```python
from build123d import *
from build123d.topology import SkipClean

# Parameters (mm, degrees)
SKETCH2_R           = 9.525
EXTRUDE1_DEPTH      = 17.526
SKETCH15_R          = 11.1125
BOSS_EXTRUDE1_DEPTH = 18.9865
SKETCH16_R          = 4.9657
CUT_EXTRUDE1_DEPTH  = 40.750949281
SKETCH20_R          = 11.1125
BOSS_EXTRUDE2_DEPTH = 18.9865
SKETCH22_R          = 10.668
BOSS_EXTRUDE3_DEPTH = 17.12976
BOSS_EXTRUDE3_TAPER = 1.75
CHAMFER1_SIZE       = 1.360714286
CHAMFER1_SIZE_2     = 1.404253042
SKETCH25_R          = 10.668
BOSS_EXTRUDE4_DEPTH = 17.12976
BOSS_EXTRUDE4_DRAFT = -15
SKETCH28_R          = 7.978385455
CUT_EXTRUDE6_DEPTH  = 17.12976
FILLET1_R           = 0.762
CIRPATTERN1_COUNT   = 2
CIRPATTERN1_ANGLE   = 180
SKETCH26_R          = 4.9657
CUT_EXTRUDE4_DEPTH  = 83.22239678
SKETCH29_R          = 4.9657
CUT_EXTRUDE7_DEPTH  = 53.545547444


with BuildPart() as part:
    # Sketch2 → Extrude1 (new body)
    with BuildSketch(Plane(origin=(-36.5125, 0, 0), x_dir=(0, 0, -1), z_dir=(1, 0, 0))):
        Circle(SKETCH2_R)
    extrude(amount=EXTRUDE1_DEPTH)

    # Sketch5 → Cut-Revolve1 (revolve, cut)
    with BuildSketch(Plane.XY):
        Polygon((-32.818891687, 8.493888504), (-29.643891687, 8.493888504), (-28.612780191, 9.525), (-36.5125, 9.525), (-36.5125, 5.710555), align=None)
        Polygon((-18.9865, 8.493888504), (-20.574, 8.493888504), (-21.605111496, 9.525), (-18.9865, 9.525), align=None)
    revolve(axis=Axis((0, 0, 0), (-1, 0, 0)), mode=Mode.SUBTRACT)

    # Sketch15 → Boss-Extrude1 (add)
    with BuildSketch(Plane(origin=(-18.9865, 0, 0), x_dir=(0, 0, -1), z_dir=(1, 0, 0))):
        Circle(SKETCH15_R)
    extrude(amount=BOSS_EXTRUDE1_DEPTH)

    # Sketch16 → Cut-Extrude1 (cut, through all)
    with BuildSketch(Plane(origin=(0, 0, 0), x_dir=(0, 0, -1), z_dir=(1, 0, 0))):
        Circle(SKETCH16_R)
    extrude(amount=-CUT_EXTRUDE1_DEPTH, mode=Mode.SUBTRACT)

    # Fillet1
    fillet1_edges = [part.edges().sort_by_distance(p)[0] for p in [
        (-18.9865, 0, 11.1125),
    ]]
    fillet(fillet1_edges, radius=FILLET1_R)


with BuildPart() as body_2:
    # Sketch20 → Boss-Extrude2 (new body)
    with BuildSketch(Plane(origin=(0, 18.9865, 0), x_dir=(-1, 0, 0), z_dir=(0, 1, 0))):
        with Locations(Location((0, 0, 0), (0, 0, 90))):
            Circle(SKETCH20_R)
    extrude(amount=-BOSS_EXTRUDE2_DEPTH)


with BuildPart() as body_3:
    # Sketch22 → Boss-Extrude3 (new body)
    with BuildSketch(Plane(origin=(0, 18.9865, 0), x_dir=(-1, 0, 0), z_dir=(0, 1, 0))):
        Circle(SKETCH22_R)
    extrude(amount=BOSS_EXTRUDE3_DEPTH, taper=BOSS_EXTRUDE3_TAPER)

    # Chamfer1
    # the kernel refuses this chamfer: 1.404253042, 1.360714286 mm, written as the material it takes off along each edge
    with BuildSketch(Plane(origin=(0, 36.11626, 0), x_dir=(-1, 0, 0), z_dir=(0, 0, 1))) as chamfer1_piece_1:
        Polygon((10.144638497 + CHAMFER1_SIZE * 0.0305385132034, CHAMFER1_SIZE * 0.999533590627), (10.144638497 - CHAMFER1_SIZE_2, 0), (10.144638497, 0), align=None)
    revolve(axis=Axis((0, 36.11626, 0), (0, -1, 0)), mode=Mode.SUBTRACT)


with BuildPart() as boss_extrude4_tool:
    # Sketch25 → Boss-Extrude4 (with draft: the straight prism first)
    with BuildSketch(Plane.XZ.offset(-18.9865)):
        Circle(SKETCH25_R)
    extrude(amount=-BOSS_EXTRUDE4_DEPTH)
    # Boss-Extrude4: the draft: its side faces are tilted about the plane it starts from
    boss_extrude4_sides = [boss_extrude4_tool.faces().sort_by_distance(p)[0] for p in [
        (-10.668, 27.55138, 0),
    ]]
    draft(boss_extrude4_sides, Plane.XZ.offset(-18.9865), BOSS_EXTRUDE4_DRAFT)


with BuildPart() as body_3_1:
    add(body_3.part)

    # Boss-Extrude4: add boss_extrude4_tool
    add(boss_extrude4_tool.part)

    # Sketch28 → Cut-Extrude6 (cut)
    with BuildSketch(Plane(origin=(0, 36.11626, 0), x_dir=(1, 0, 0), z_dir=(0, 1, 0))):
        with Locations(Location((0, 0, 0), (0, 0, 270))):
            Circle(SKETCH28_R)
    extrude(amount=-CUT_EXTRUDE6_DEPTH, mode=Mode.SUBTRACT)


with BuildPart() as cirpattern1_1:
    # CirPattern1: pattern copy
    add(part.part.rotate(Axis((0, 0, 12.651043997), (0, 0, -1)), 1 * CIRPATTERN1_ANGLE / (CIRPATTERN1_COUNT - 1)))


with BuildPart() as part_1:
    add(part.part)

    # Combine2: union body 3, body 2, CirPattern1_1
    add(body_3_1.part)
    add(body_2.part)
    add(cirpattern1_1.part)

    # Sketch30 → Revolve1 (revolve)
    with SkipClean():  # the faces are left unmerged after this step: merging them gives an invalid solid
        with BuildSketch(Plane.XY, mode=Mode.PRIVATE) as revolve1_sk:
            with BuildLine():
                Line((0, 18.9865), (0, 9.49325))
                ThreePointArc((0, 9.49325), (-5.981989992, 13.352586812), (-10.922, 18.4785))
                Line((-10.922, 18.4785), (-10.922, 18.9865))
                Line((-10.922, 18.9865), (0, 18.9865))
            make_face()
        revolve(revolve1_sk.sketch.rotate(Axis((0, 18.9865, 0), (0, -1, 0)), 270), axis=Axis((0, 18.9865, 0), (0, -1, 0)))

    # Sketch26 → Cut-Extrude4 (cut, through all)
    with SkipClean():  # the faces are left unmerged after this step: merging them gives an invalid solid
        with BuildSketch(Plane.ZY.offset(36.5125)):
            with Locations(Location((0, 0, 0), (0, 0, 180))):
                Circle(SKETCH26_R)
        extrude(amount=-CUT_EXTRUDE4_DEPTH, mode=Mode.SUBTRACT)

    # Sketch29 → Cut-Extrude7 (cut, through all)
    with SkipClean():  # the faces are left unmerged after this step: merging them gives an invalid solid
        with BuildSketch(Plane(origin=(0, 0, 0), x_dir=(1, 0, 0), z_dir=(0, 1, 0))):
            with Locations(Location((0, 0, 0), (0, 0, 270))):
                Circle(SKETCH29_R)
        extrude(amount=CUT_EXTRUDE7_DEPTH, mode=Mode.SUBTRACT)


solid = part_1.part
```
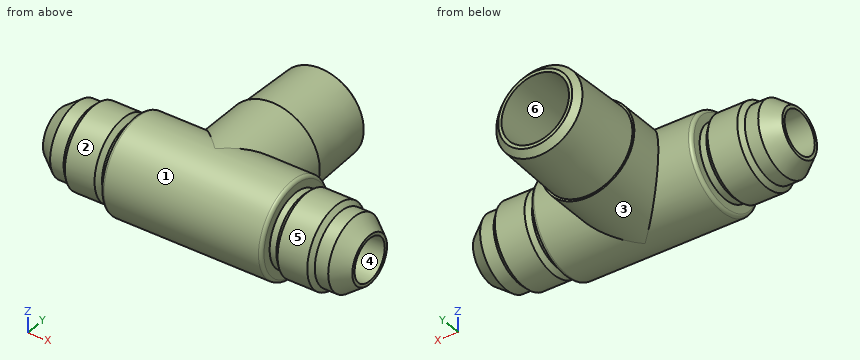
Source: CAD feature listing. Evaluate the final solid. Frame: model axes, mm. Face numbers are marked on the shaded views. A direction names the side the tool comes from. Give positions to 0.01 mm unless a question says otherwise; leave off trailing zeros. Write each loop counter-clockwise with the first axis right and the second up, starting at its lowest first coordinate (ties: lowest second). Pieces come first, ordered by that corner, then holes.
1. Pull-direction query (Y, two-part tool) for the marked faces 4, 5 and 6; classes: +Y half, -Y half, draft (parallel to the pull), parting line (faces both ways), or undercut.
2. Section query C-C (x = 15). Return the cut outline in (y, z) (1 decimal).
3. Section query A-A (x = 0). Return the cut outline in (y, z) (1 decimal).
4. Access query for the marked faces 1, 2 and 3. Directions: +Z, -Z, +X, -X, +Y, -Y. A direction counts if a zero-diameter tool reaches every point of the face in a straight line with its end or side. Return the directions, or none.
5. Section query B-B (z = 0). Count the separate pieces of the cut face and the enclosed holes in it, then the cut area to 3 significant figures.
6. First-contact query: pin 1 (2 mm diameter, centred on y = 28, z = 2.5, fed in from -X); pin 2 (2 mm diameter, centred on x = 16.5, z = -1, fed in from +Y); pin 3 (1 mm diameter, centred on x = -5.5, z = 1.5, fed in from +Y). Flat tips, straight axial feed; report the tip coordinate or a pass-through.
7. Material intervals for line 1 along X through (y, z) = (13.25, 0), sorted ascending.
Output values:
1. face 4: undercut
1. face 5: parting line
1. face 6: draft
2. outline: circle Ø22.2 at (0, 0); hole circle Ø9.9 at (0, 0)
3. outline: (0, -11.1) - (19, -11.1) - (19, -10.7) - (34.8, -10.2) - (36.1, -8.7) - (36.1, -8) - (19, -8) - (19, -5) - (0, -5) arc R5 cw to (0, 5) - (19, 5) - (19, 8) - (36.1, 8) - (36.1, 8.7) - (34.8, 10.2) - (19, 10.7) - (19, 11.1) - (0, 11.1) arc R11.1 ccw to start
4. face 1: none
4. face 2: -X
4. face 3: +Y
5. separate pieces: 3
5. enclosed holes: 0
5. area: 843 mm2
6. pin 1: stops at x = -10.29
6. pin 2: stops at y = 11.11
6. pin 3: stops at y = 18.99
7. line 1: x = -11.11 to -4.97, 4.97 to 11.11
